```python
from build123d import *

# Parameters (mm, degrees)
BOSS_EXTRUDE6_DEPTH = 19.05
CUT_EXTRUDE2_DEPTH  = 17.05
FILLET2_R           = 3
FILLET1_R           = 1


with BuildPart() as part:
    # Sketch3 → Boss-Extrude6 (new body)
    with BuildSketch(Plane.XY):
        with BuildLine():
            Line((0, 0), (35, 0))
            ThreePointArc((35, 0), (-34.548087395, 5.606215958), (33.204019579, -11.067659364))
            Line((33.204019579, -11.067659364), (16.658538837, -11.067659364))
            ThreePointArc((16.658538837, -11.067659364), (-5.780537313, -19.146419727), (-20, 0))
            Line((-20, 0), (0, 0))
        make_face()
        with BuildLine():
            Line((-17.320508076, 10), (17.320508076, 10))
            ThreePointArc((17.320508076, 10), (0, 20), (-17.320508076, 10))
        make_face(mode=Mode.SUBTRACT)
    extrude(amount=BOSS_EXTRUDE6_DEPTH)

    # Sketch6 → Cut-Extrude2 (cut)
    with BuildSketch(Plane.XY.offset(19.05)):
        with BuildLine():
            Line((29.532501069, -13.567659364), (17.949056225, -13.567659364))
            ThreePointArc((17.949056225, -13.567659364), (-8.331147877, -20.900764939), (-22.360679775, 2.5))
            Line((-22.360679775, 2.5), (20, 2.5))
            Line((20, 2.5), (32.403703492, 2.5))
            ThreePointArc((32.403703492, 2.5), (-31.993214565, 5.717011614), (29.532501069, -13.567659364))
        make_face()
        with BuildLine():
            Line((21.213203436, 7.5), (-21.213203436, 7.5))
            ThreePointArc((-21.213203436, 7.5), (0, 22.5), (21.213203436, 7.5))
        make_face(mode=Mode.SUBTRACT)
    extrude(amount=-CUT_EXTRUDE2_DEPTH, mode=Mode.SUBTRACT)

    # Fillet2
    fillet2_edges = [part.edges().sort_by_distance(p)[0] for p in [
        (29.532501069, -13.567659364, 10.525),
        (32.403703492, 2.5, 10.525),
        (33.204019579, -11.067659364, 9.525),
        (35, 0, 9.525),
    ]]
    fillet(fillet2_edges, radius=FILLET2_R)

    # Fillet1
    fillet1_edges = [part.edges().sort_by_distance(p)[0] for p in [
        (3.311036859, 2.5, 2),
        (-8.331147877, -20.900764939, 2),
        (-22.360679775, 2.5, 10.525),
        (17.949056225, -13.567659364, 10.525),
        (0, 7.5, 2),
        (0, 22.5, 2),
        (21.213203436, 7.5, 10.525),
        (-21.213203436, 7.5, 10.525),
        (-31.823448952, 6.596824754, 2),
        (21.178653063, -13.567659364, 2),
        (27.059149761, -15.16312032, 2),
        (31.293377445, 3.586621588, 2),
    ]]
    fillet(fillet1_edges, radius=FILLET1_R)


solid = part.part
```
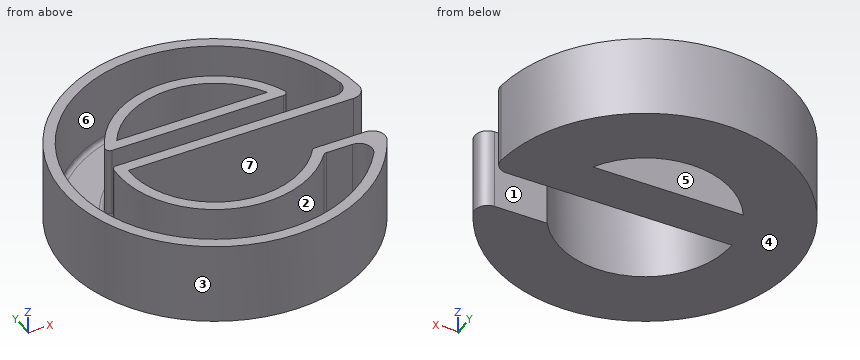
Can you work these out from the model? Positions are in its coordinate system, mm. Face numbers are marked on the shaded views. A direction names the side the tool comes from. Give positions to 0.01 mm unless a question says otherwise; leave off trailing zeros. Loops run counter-clockwise (first coordinate to the right, second up) from the corner with the lowest first, then second, coordinate; pieces in that order, holes last. Notation, with made-up numbers: M -33,3.25 L 25,3.25 A15 cw 25,32.25 Z; hole C -33.75,-29.5 d8. An arc over 180 degrees is marked long. Use one line per item in the form item = value. Start each with the question number.
(1) I'm going to push flat-ended pins straight in: P1, Ø1.5, axis at x = -14, z = 8.5, coming from the +Y side (3 decimals); P2, Ø1.5, axis at x = 16, z = 9, coming from the -Y side; P3, Ø1.8, axis at x = 21, z = 15, coming from the -Y side; P4, Ø6, axis at x = 26.5, y = -4.5, coming from the +Z side. Where does each tip first touch, or does it pass through?
(2) I want a section at B-B, the plane x = 0. State how many separate pieces and enclosed holes the cut face has, and give its area (3 significant figures).
(3) Thinking about a two-plate mould opening in X: for the marked faces 1, 2 and 3, which applies, released by +X, released by -X, zero draft, split by the parting line, or undercut?
(4) I want a section at A-A, the plane z = 8.5. Write out the boundary of the cut face in (x, y), and give its area (3 significant figures).
(5) On a 3-axis mill with a long thin cutter (end or side, diameter ignored), from which of +Z, -Z, +X, -X, +Y, -Y can I reach the whole of each face in a straight line? I mean the marked faces 4, 5, 6 and 7. Say none if no direction works.
(6) Please list where these lines run through material, in increasing order: line 1 (Y direction, x = 0, z = 15.5); line 2 (Y direction, x = 15, z = 4.5); line 3 (Y direction, x = 27.5, z = 16.25).
Worked out:
q1.P1 = 32.395
q1.P2 = -31.5
q1.P3 = -28.65
q1.P4 = through
q2.separate_pieces = 3
q2.enclosed_holes = 0
q2.area = 337 mm²
q3.face_1 = zero draft
q3.face_2 = undercut
q3.face_3 = split by the parting line
q4.outline = M -20.67,8.9 A1 ccw -19.75,7.5 L 19.75,7.5 A1 ccw 20.67,8.9 A22.5 ccw Z; M -20,0 L 31.86,0 A3 ccw 34.85,3.28 A35 ccw long 31.44,-15.39 A3 ccw 28.74,-11.07 L 16.66,-11.07 A20 cw Z; hole M -22.45,1.57 A1 cw -21.45,2.5 L 28.98,2.5 A3 ccw 31.93,6.06 A32.5 ccw long 26.89,-18.25 A3 ccw 24.41,-13.57 L 18.44,-13.57 A1 ccw 17.66,-13.95 A22.5 cw Z; hole M -17.32,10 L 17.32,10 A20 ccw Z
q4.area = 1,020 mm²
q5.face_4 = -Z, +X, -X, +Y, -Y
q5.face_5 = +Z, -Z
q5.face_6 = +Z
q5.face_7 = +Z, -Z, +X
q6.line_1 = -35 to -32.5, -22.5 to -20, 0 to 2.5, 7.5 to 10, 20 to 22.5, 32.5 to 35
q6.line_2 = -31.62 to -28.83, -16.77 to -13.23, 0 to 2.5, 7.5 to 10, 13.23 to 16.77, 28.83 to 31.62
q6.line_3 = -21.65 to -11.07, 0 to 2.5, 17.32 to 21.65
